Verification items for the finished model (mm, model axes). Coordinates: 2 decimals unless noted, no trailing zeros. Loops run counter-clockwise (first coordinate to the right, second up) from the corner with the lowest first, then second, coordinate; pieces in that order, holes last. Notation, with made-up numbers: (1.5, 37.5) -> (50.5, 37.5) arc R16 ccw to (50.5, 61.5) -> close; hole circle Ø8 at (3, 21). An arc over 180 degrees is marked (long way). Use CSV: the item, a comma, the result in double quotes. Start each with the question number.
```python
from build123d import *


with BuildPart() as part:
    # Çizim1 → Döndür1 (revolve)
    with BuildSketch(Plane.XY):
        Polygon((14.556330182, -0.000478985), (14.556330182, 4.716980057), (9.797530392, 4.716980057), (9.797530392, -0.000478985), (11.332803263, -0.000478985), (12.01520523, 2.781914958), (12.530984141, 2.810062352), (13.691331204, -0.000478985), align=None)
    revolve(axis=Axis((0, 0, 0), (4.8888323348204376e-05, 0.9999999988049659, 0)))


solid = part.part
```
1. Cross-section at B-B, the plane y = 2.25. State how many separate pieces and enclosed holes the cut face has, plus the area to 3 significant figures.
2. Cross-section at A-A, the plane z = 0. Record the boundary of the cut face in (x, y), plus the area to 3 significant figures.
3. Depth check by flat-ended pin: pin 1 (1 mm diameter, centred on y = 0.5, z = 5, fed in from -X); pin 2 (1.5 mm diameter, centred on x = -10, y = 1, fed in from -Z); pin 3 (2 mm diameter, centred on x = 1.5, y = 2.5, fed in from +Z). Enter the tip coordinate at first touch or a pass-through.
4. Scan lines: line 1 (X direction, y = 1.85, z = -3.25); line 2 (Z direction, x = -8.25, y = 1.65); line 3 (Z direction, x = -7.75, y = 0.8). Record each from-to range of solid material in increasing order.
5. Release check for a two-part mould opening along Z. For faces 1 (the cylindrical face through (-3.2, 2.4, 14.2)), 2 (the conical face through (-2.466, 0.174, 11.105)), 3 (the conical face through (9.566, 4.717, -3.012)), 4 (the conical face through (-2.732, 2.635, 12.304)) record: released by +Z, released by -Z, zero draft, split by the parting line, or undercut.
Solution:
1,separate pieces,"2"
1,enclosed holes,"2"
1,area,"296 mm2"
2,outline,"(-14.56, 0) -> (-13.69, 0) -> (-12.53, 2.81) -> (-12.01, 2.78) -> (-11.33, 0) -> (-9.8, 0) -> (-9.8, 4.72) -> (-14.56, 4.72) -> close; (9.8, 0) -> (11.33, 0) -> (12.02, 2.78) -> (12.53, 2.81) -> (13.69, 0) -> (14.56, 0) -> (14.56, 4.72) -> (9.8, 4.72) -> close"
2,area,"36.9 mm2"
3,pin 1,"stops at x = -13.84"
3,pin 2,"stops at z = -11.24"
3,pin 3,"stops at z = 14.55"
4,line 1,"x = -14.19 to -12.51, -11.33 to -9.24, 9.24 to 11.33, 12.51 to 14.19"
4,line 2,"z = -11.99 to -10.06, -8.35 to -5.28, 5.28 to 8.35, 10.06 to 11.99"
4,line 3,"z = -12.32 to -10.88, -8.54 to -5.99, 5.99 to 8.54, 10.88 to 12.32"
5,face 1,"split by the parting line"
5,face 2,"undercut"
5,face 3,"zero draft"
5,face 4,"undercut"
